from build123d import *

# Parameters (mm, degrees)
SKETCH1_W                 = 95.25
SKETCH1_H                 = 38.1
SKETCH1_R                 = 7.5
SKETCH1_R_2               = 10
BOSS_EXTRUDE1_DEPTH       = 5.8
CBORE_FOR_M3_SHCS1_DEPTH  = 5.8
CUT_EXTRUDE1_DEPTH        = 103.751216538
FILLET1_R                 = 3.175
F_4_CLEARANCE_HOLE1_D     = 2.9464
F_4_CLEARANCE_HOLE1_DEPTH = 5.8
F_4_CLEARANCE_HOLE1_TIP   = 0.885187864
SKETCH11_R                = 0.79375
CUT_EXTRUDE2_DEPTH        = 103.751216538
FILLET2_R                 = 3.175
M3X0_5_TAPPED_HOLE1_D     = 2.5
M3X0_5_TAPPED_HOLE1_DEPTH = 7.5
M3X0_5_TAPPED_HOLE1_TIP   = 0.751075774
M3X0_5_TAPPED_HOLE2_D     = 2.5
M3X0_5_TAPPED_HOLE2_DEPTH = 8.5
M3X0_5_TAPPED_HOLE2_TIP   = 0.751075774
SKETCH17_R                = 0.79375
CUT_EXTRUDE3_DEPTH        = 103.751216538


# Read off the part's stored shape, not the designer's step: CBORE for M3 SHCS1
with BuildPart() as part:
    # Sketch1 → Boss-Extrude1 (new body)
    with BuildSketch(Plane.XY):
        with Locations((47.625, 19.05)):
            Rectangle(SKETCH1_W, SKETCH1_H)
        with Locations((73.025, 19.05)):
            Circle(SKETCH1_R, mode=Mode.SUBTRACT)
        with Locations((27.263471398, 25.4)):
            Circle(SKETCH1_R_2, mode=Mode.SUBTRACT)
    extrude(amount=BOSS_EXTRUDE1_DEPTH)

    # CBORE for M3 SHCS1 outline → CBORE for M3 SHCS1 (cut)
    with BuildSketch(Plane.XY):
        with BuildLine():
            ThreePointArc((34.571649716, 18.574274422), (32.263471398, 16.739745962), (29.520633989, 15.658069132))
            ThreePointArc((29.520633989, 15.658069132), (34.388471398, 13.059137996), (34.571649716, 18.574274422))
        make_face()
        with BuildLine():
            ThreePointArc((19.95529308, 18.574274422), (20.138471398, 13.059137996), (25.006308807, 15.658069132))
            ThreePointArc((25.006308807, 15.658069132), (22.263471398, 16.739745962), (19.95529308, 18.574274422))
        make_face()
        with BuildLine():
            ThreePointArc((36.828812307, 28.31620529), (37.263471398, 25.4), (36.828812307, 22.48379471))
            ThreePointArc((36.828812307, 22.48379471), (41.513471398, 25.4), (36.828812307, 28.31620529))
        make_face()
        with BuildLine():
            ThreePointArc((17.698130489, 28.31620529), (13.013471398, 25.4), (17.698130489, 22.48379471))
            ThreePointArc((17.698130489, 22.48379471), (17.263471398, 25.4), (17.698130489, 28.31620529))
        make_face()
        with BuildLine():
            ThreePointArc((19.95529308, 32.225725578), (27.263471398, 35.4), (34.571649716, 32.225725578))
            ThreePointArc((34.571649716, 32.225725578), (35.957138985, 35.528763749), (33.463469839, 38.1))
            Line((33.463469839, 38.1), (21.063472957, 38.1))
            ThreePointArc((21.063472957, 38.1), (18.56980381, 35.528763749), (19.95529308, 32.225725578))
        make_face()
    extrude(amount=CBORE_FOR_M3_SHCS1_DEPTH, mode=Mode.SUBTRACT)

    # Sketch3 → Cut-Extrude1 (cut, through all)
    with BuildSketch(Plane.XY.offset(5.8)):
        with BuildLine():
            Line((50.731096487, 10.325758959), (41.37076894, 8.562270029))
            ThreePointArc((41.37076894, 8.562270029), (38.838489401, 4.854331203), (42.546428227, 2.322051664))
            Line((42.546428227, 2.322051664), (51.906755774, 4.085540594))
            ThreePointArc((51.906755774, 4.085540594), (54.439035313, 7.79347942), (50.731096487, 10.325758959))
        make_face()
    extrude(amount=-CUT_EXTRUDE1_DEPTH, mode=Mode.SUBTRACT)

    # Fillet1
    fillet1_edges = [part.edges().sort_by_distance(p)[0] for p in [
        (0, 0, 2.9),
        (0, 38.1, 2.9),
        (95.25, 38.1, 2.9),
        (95.25, 0, 2.9),
    ]]
    fillet(fillet1_edges, radius=FILLET1_R)

    # #4 Clearance Hole1
    with Locations(Plane.XY.offset(5.8)):
        with Locations((4.7625, 33.3375), (4.7625, 4.7625), (23.8125, 4.7625), (90.4875, 4.7625), (90.4875, 33.3375)):
            Hole(F_4_CLEARANCE_HOLE1_D / 2, depth=F_4_CLEARANCE_HOLE1_DEPTH)
            with Locations((0, 0, -(F_4_CLEARANCE_HOLE1_DEPTH + F_4_CLEARANCE_HOLE1_TIP / 2))):  # 118° drill point
                Cone(0, F_4_CLEARANCE_HOLE1_D / 2, F_4_CLEARANCE_HOLE1_TIP, mode=Mode.SUBTRACT)

    # Sketch11 → Cut-Extrude2 (cut, through all)
    with BuildSketch(Plane.XY.offset(5.8)):
        with Locations((4.7625, 19.05)):
            Circle(SKETCH11_R)
        with Locations((14.2875, 4.7625)):
            Circle(SKETCH11_R)
        with Locations((57.15, 4.7625)):
            Circle(SKETCH11_R)
        with Locations((90.4875, 19.05)):
            Circle(SKETCH11_R)
    extrude(amount=-CUT_EXTRUDE2_DEPTH, mode=Mode.SUBTRACT)

    # Fillet2
    fillet2_edges = [part.edges().sort_by_distance(p)[0] for p in [
        (33.463469839, 38.1, 2.9),
        (21.063472957, 38.1, 2.9),
    ]]
    fillet(fillet2_edges, radius=FILLET2_R)

    # M3x0.5 Tapped Hole1
    with Locations(Plane.XY.offset(5.8)):
        with Locations((11.388471398, 34.925), (43.138471398, 34.925), (43.138471398, 15.875), (11.388471398, 15.875)):
            Hole(M3X0_5_TAPPED_HOLE1_D / 2, depth=M3X0_5_TAPPED_HOLE1_DEPTH)
            with Locations((0, 0, -(M3X0_5_TAPPED_HOLE1_DEPTH + M3X0_5_TAPPED_HOLE1_TIP / 2))):  # 118° drill point
                Cone(0, M3X0_5_TAPPED_HOLE1_D / 2, M3X0_5_TAPPED_HOLE1_TIP, mode=Mode.SUBTRACT)

    # M3x0.5 Tapped Hole2
    with Locations(Plane.XY.offset(5.8)):
        with Locations((64.606009886, 27.468990114), (81.443990114, 27.468990114), (81.443990114, 10.631009886), (64.606009886, 10.631009886)):
            Hole(M3X0_5_TAPPED_HOLE2_D / 2, depth=M3X0_5_TAPPED_HOLE2_DEPTH)
            with Locations((0, 0, -(M3X0_5_TAPPED_HOLE2_DEPTH + M3X0_5_TAPPED_HOLE2_TIP / 2))):  # 118° drill point
                Cone(0, M3X0_5_TAPPED_HOLE2_D / 2, M3X0_5_TAPPED_HOLE2_TIP, mode=Mode.SUBTRACT)

    # Sketch17 → Cut-Extrude3 (cut, through all)
    with BuildSketch(Plane.XY.offset(5.8)):
        with Locations((61.11875, 19.05)):
            Circle(SKETCH17_R)
        with Locations((73.025, 7.14375)):
            Circle(SKETCH17_R)
        with Locations((84.93125, 19.05)):
            Circle(SKETCH17_R)
        with Locations((73.025, 30.95625)):
            Circle(SKETCH17_R)
    extrude(amount=-CUT_EXTRUDE3_DEPTH, mode=Mode.SUBTRACT)


solid = part.part
Can you work these out from the model? Positions are in its coordinate system, mm. A direction names the side the tool comes from. Coordinates: 2 decimals unless noted, no trailing zeros. Write each loop counter-clockwise with the first axis right and the second up, starting at its lowest first coordinate (ties: lowest second). Pieces come first, ordered by that corner, then holes. Notation, with made-up numbers: (-23, -33) -> (30, -33) arc R31 ccw to (30, -5) -> close; hole circle Ø8 at (-33.5, 50.25). An arc over 180 degrees is marked (long way). Write each question's results on one line, items separated by ' | '. Start each with the question number.
Item 1: Thinking about a two-plate mould opening in X: for faces 1 (the flat face through (47, 19, 0)), 2 (the cylindrical face through (0.91, 37.15, 2.94)), 3 (the cylindrical face through (43.301, 36.164, 2.859)), which applies, released by +X, released by -X, zero draft, split by the parting line, or undercut?
Item 2: If we section it at B-B, the plane z = 4.9: Count the separate pieces of the cut face and the enclosed holes in it, and give its area (3 significant figures).
Item 3: Please list where these lines run through material, in increasing order: probe 1 along X at (y, z) = (35, 0.4); probe 2 along Y at (x, z) = (12.5, 0.45); probe 3 along X at (y, z) = (31.5, 4.25).
Item 4: If we section it at A-A, the plane x = 75: Write out the boundary of the cut face in (y, z), and give its area (3 significant figures).
Item 5: On a 3-axis mill with a long thin cutter (end or side, diameter ignored), from which of +Z, -Z, +X, -X, +Y, -Y can I reach the whole of each face in a straight line? I mean faces 4 (the cylindrical face through (18.886, 33.415, 2.859)), 5 (the cylindrical face through (35.94, 30.37, 2.86)), 6 (the flat face through (65, 38.1, 3)). Say none if no direction works.
Answer block:
1) face 1: zero draft | face 2: released by -X | face 3: undercut
2) separate pieces: 1 | enclosed holes: 23 | area: 2,780 mm²
3) probe 1: 0 to 10.14, 12.64 to 18.51, 36.01 to 41.89, 44.39 to 95.25 | probe 2: 0 to 15.3, 16.45 to 34.35, 35.5 to 38.1 | probe 3: 0 to 19.34, 35.19 to 72.45, 73.6 to 95.25
4) outline: (0, 0) -> (11.81, 0) -> (11.81, 5.8) -> (0, 5.8) -> close; (26.29, 0) -> (38.1, 0) -> (38.1, 5.8) -> (26.29, 5.8) -> close | area: 137 mm²
5) face 4: +Z, -Z, +Y | face 5: +Z, -Z | face 6: +Z, -Z, +X, -X, +Y
